Work out the finished part from the listing and answer in its coordinate system (mm). Face numbers are marked on the shaded views. A direction names the side the tool comes from. Give positions to 0.01 mm unless a question says otherwise; leave off trailing zeros. Write each loop counter-clockwise with the first axis right and the second up, starting at its lowest first coordinate (ties: lowest second). Pieces come first, ordered by that corner, then holes.
1) A tool of negligible diameter and unlimited length cuts with its end or side. For the marked faces 1, 2 and 3, from which of +Z, -Z, +X, -X, +Y, -Y can it reach the whole face along a straight path? Write none if from no direction.
2) Straight lines are drawn through the part: probe 1 along X at (y, z) = (151, -112); probe 2 along Y at (x, z) = (725, 42); probe 3 along Y at (x, z) = (633, 185). For each, find the intervals that lie inside material, in ascending order.
3) Find section D-D (y = 142). Determine the outline of the cut face in (x, z).
4) Find section A-A (z = -145). Determine the outline of the cut face in (x, y), plus the area to 4 significant figures.
5) Find section B-B (x = 771.5). Determine the outline of the cut face in (y, z), plus the area to 3 significant figures.
6) Find section C-C (z = -219). Determine the outline of the cut face in (x, y), plus the area to 3 significant figures.
7) Given pin 1 Ø10 at (x, y) = (527, 11) entering from +Z, flat-ended and moving along its own axis, determine where the tip first touches the part or whether it passes through.
8) Determine the mould class of the marked faces 4, 5 and 6 for opening direction X: pulls with the +X half, pulls with the -X half, needs draft (parallel to the pull), parting line crosses it, or undercut.
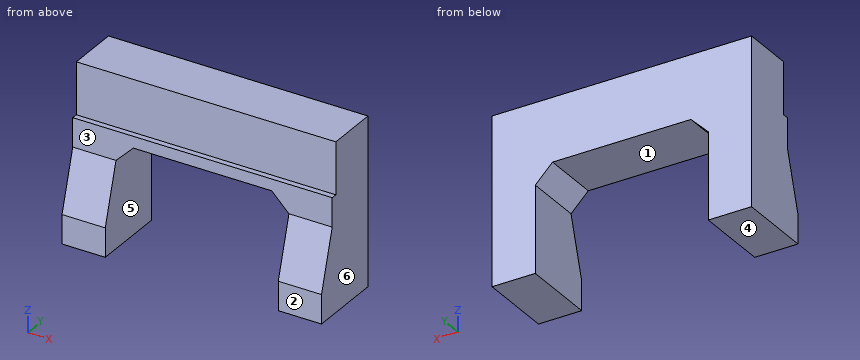
```python
from build123d import *

# Parameters (mm, degrees)
SKETCH_W          = 200
SKETCH_H          = 100
SKETCH_W_2        = 180
SKETCH_H_2        = 150
SKETCH_H_3        = 30
PAD_DEPTH         = 900
POCKET_DEPTH      = 200.001
POCKET_DEPTH_BACK = -60.001
SKETCH002_W       = 20
SKETCH002_H       = 30
POCKET001_DEPTH   = 900.001


with BuildPart() as part:
    # Sketch → Pad (new body)
    with BuildSketch(Plane.YZ):
        with Locations((100, 50)):
            Rectangle(SKETCH_W, SKETCH_H)
        with Locations((110, 175)):
            Rectangle(SKETCH_W_2, SKETCH_H_2)
        with Locations((100, 265)):
            Rectangle(SKETCH_W, SKETCH_H_3)
        Polygon((0, 0), (200, 0), (200, -300), (-60, -300), (-60, -200), align=None)
    extrude(amount=PAD_DEPTH)

    # Sketch001 (on Face6 of Pad) → Pocket (cut, two sides)
    with BuildSketch(Plane(origin=(0, 0, 0), x_dir=(0, 0, -1), z_dir=(0, -1, 0))) as pocket_sk:
        Polygon((0, 150), (494.350739, 150), (494.350739, 750), (0, 750), (-60, 690), (-60, 210), align=None)
    extrude(amount=-POCKET_DEPTH, mode=Mode.SUBTRACT)
    extrude(pocket_sk.sketch, amount=-POCKET_DEPTH_BACK, mode=Mode.SUBTRACT)

    # Sketch002 (on Face5 of Pocket) → Pocket001 (cut, through all)
    with BuildSketch(Plane.YZ.offset(900)):
        with Locations((10, 265)):
            Rectangle(SKETCH002_W, SKETCH002_H)
    extrude(amount=-POCKET001_DEPTH, mode=Mode.SUBTRACT)


solid = part.part
```
Results:
1. face 1: -Z, +Y, -Y
1. face 2: +Z, -Z, +X, -X, -Y
1. face 3: +Z, +X, -X, -Y
2. probe 1: x = 0 to 150, 750 to 900
2. probe 2: y = 0 to 200
2. probe 3: y = 20 to 200
3. outline: (0, -300) - (150, -300) - (150, 0) - (210, 60) - (690, 60) - (750, 0) - (750, -300) - (900, -300) - (900, 280) - (0, 280) - close
4. outline: (0, -43.5) - (150, -43.5) - (150, 200) - (0, 200) - close; (750, -43.5) - (900, -43.5) - (900, 200) - (750, 200) - close
4. area: 73,050 mm2
5. outline: (-60, -300) - (200, -300) - (200, 280) - (20, 280) - (20, 100) - (0, 100) - (0, 0) - (-60, -200) - close
5. area: 124,000 mm2
6. outline: (0, -60) - (150, -60) - (150, 200) - (0, 200) - close; (750, -60) - (900, -60) - (900, 200) - (750, 200) - close
6. area: 78,000 mm2
7. pin 1: stops at z = 100
8. face 4: needs draft
8. face 5: undercut
8. face 6: pulls with the +X half
